```python
from build123d import *

# Parameters (mm, degrees)
F0_W     = 685.8
F0_H     = 88.9
F0_R     = 3.175
F0_R_2   = 6.35
F1_DEPTH = 38.1
F2_R     = 25.4
F3_R     = 6.35


with BuildPart() as f1:
    # F0 (on Front) → F1 (new body)
    with BuildSketch(Plane.XZ):
        with Locations((176.894678, 19.006401)):
            Rectangle(F0_W, F0_H)
        with Locations((-51.705322, -6.393599)):
            Circle(F0_R, mode=Mode.SUBTRACT)
        with Locations((100.694678, -6.393599)):
            Circle(F0_R, mode=Mode.SUBTRACT)
        with Locations((-146.955322, 4.274401)):
            Circle(F0_R_2, mode=Mode.SUBTRACT)
        with Locations((253.094678, -6.393599)):
            Circle(F0_R, mode=Mode.SUBTRACT)
        with Locations((405.494678, -6.393599)):
            Circle(F0_R, mode=Mode.SUBTRACT)
        with Locations((500.744678, 4.274401)):
            Circle(F0_R_2, mode=Mode.SUBTRACT)
        with Locations((-146.955322, 33.738401)):
            Circle(F0_R_2, mode=Mode.SUBTRACT)
        with Locations((500.744678, 33.738401)):
            Circle(F0_R_2, mode=Mode.SUBTRACT)
    extrude(amount=-F1_DEPTH)

    # F2
    f2_edges = [f1.edges().sort_by_distance(p)[0] for p in [
        (519.794678, 19.05, 63.456401),
        (519.794678, 19.05, -25.443599),
        (-166.005322, 19.05, 63.456401),
        (-166.005322, 19.05, -25.443599),
    ]]
    fillet(f2_edges, radius=F2_R)

    # F3
    f3_edges = [f1.edges().sort_by_distance(p)[0] for p in [
        (176.894678, 0, 63.456401),
        (176.894678, 38.1, 63.456401),
    ]]
    fillet(f3_edges, radius=F3_R)


solid = f1.part
```
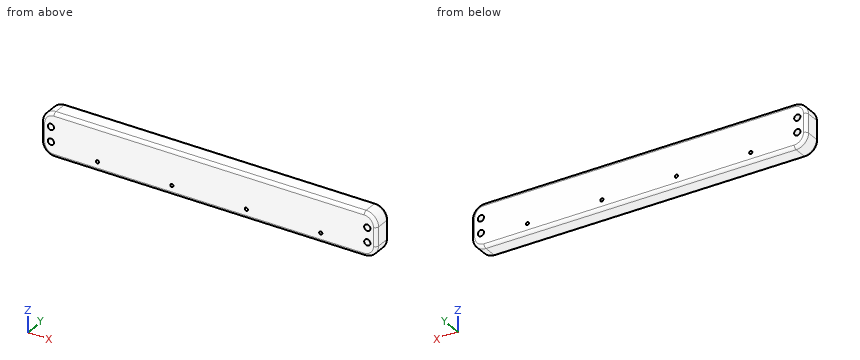
The listing builds one solid part. Answer for the finished solid, in the listing's coordinates (mm). Give positions to 0.01 mm unless a question says otherwise; leave off trailing zeros. One line per item, written item: value.
1) Find the intervals of material crossed by line 1 (X direction, y = 13.5, z = -6); line 2 (X direction, y = 3, z = 4.5); line 3 (X direction, y = 12, z = 32), in increasing order.
Reported:
line 1: x = -165.3 to -54.86, -48.55 to 97.54, 103.85 to 249.94, 256.25 to 402.34, 408.65 to 519.09
line 2: x = -165.05 to -153.3, -140.61 to 494.4, 507.09 to 518.84
line 3: x = -166.01 to -153.06, -140.85 to 494.64, 506.85 to 519.79
2) Flat-ended cylindrical pins translate along their axes: P1, Ø3, axis at y = 19, z = 41, coming from the -X side; P2, Ø1, axis at y = 30, z = -4, coming from the -X side; P3, Ø1, axis at y = 5, z = 52, coming from the +X side. Find the tip coordinate at first contact, or state that the pin passes through.
Reported:
P1: stops at x = -165.96
P2: stops at x = -165.77
P3: stops at x = 515.8
3) Find section A-A, the plane y = 22. Count the separate pieces of the cut face and the enclosed holes in it, plus the area to 3 significant figures.
Reported:
separate pieces: 1
enclosed holes: 8
area: 59,800 mm^2
